```python
from build123d import *

# Parameters (mm, degrees)
F0_R     = 1.5875
F1_DEPTH = 12.7


with BuildPart() as f1:
    # F0 (on Front) → F1 (new body)
    with BuildSketch(Plane.XZ):
        with BuildLine():
            Line((-12.238163, 28.612093), (-55.574305, 28.462326))
            ThreePointArc((-55.574305, 28.462326), (-59.292865, 24.743766), (-55.574305, 21.025206))
            Line((-55.574305, 21.025206), (-12.224796, 20.875369))
            ThreePointArc((-12.224796, 20.875369), (-8.343011, 24.73708), (-12.211425, 28.612186))
            ThreePointArc((-12.211425, 28.612186), (-12.224794, 28.612162), (-12.238163, 28.612093))
        make_face()
        with Locations((-55.574305, 24.743766)):
            Circle(F0_R, mode=Mode.SUBTRACT)
        with Locations((-12.211425, 24.743766)):
            Circle(F0_R, mode=Mode.SUBTRACT)
    extrude(amount=F1_DEPTH)


solid = f1.part
```
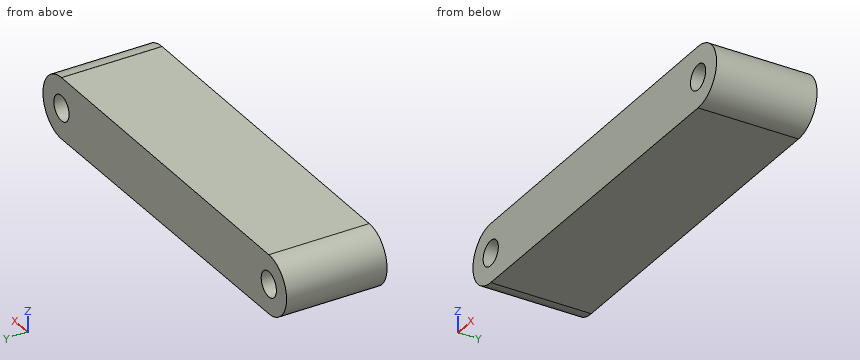
Source: CAD feature listing. Evaluate the final solid. Frame: model axes, mm. Give positions to 0.01 mm unless a question says otherwise; leave off trailing zeros. Order: outer loops, then holes, each group sorted by start corner. A loop starts at its lowest first (then second) coordinate and runs counter-clockwise, first axis right, second up.
(1) Contact query for flat-ended pins moving along their axis: P1, Ø4, axis at y = -9, z = 22, coming from the +X side; P2, Ø1.9, axis at x = -55.57, z = 24.74, coming from the +Y side; P3, Ø1.5, axis at y = -3.5, z = 22.5, coming from the +X side; P4, Ø1, axis at y = -7, z = 28, coming from the -X side. Output: stop coordinate, or through.
(2) Section query A-A (z = 23.75). Return the cut outline in (x, y), plus the area to 3 significant figures.
(3) Section query D-D (z = 28). Return the cut outline in (x, y).
(4) Section query B-B (y = -4.5). State how many separate pieces and enclosed holes the cut face has, plus the area to 3 significant figures.
(5) Material intervals for line 1 along X through (y, z) = (-6.5, 24.75); line 2 along X through (y, z) = (-9.5, 26); line 3 along Z through (x, y) = (-11, -7), sorted ascending.
(6) Section query C-C (x = -32.5). Return the cut outline in (y, z), plus the area to 3 significant figures.
Outcome:
1. P1: stops at x = -8.42
1. P2: passes through
1. P3: stops at x = -8.64
1. P4: stops at x = -58.07
2. outline: (-59.16, -12.7) - (-56.81, -12.7) - (-56.81, 0) - (-59.16, 0) - close; (-54.34, -12.7) - (-13.45, -12.7) - (-13.45, 0) - (-54.34, 0) - close; (-10.97, -12.7) - (-8.47, -12.7) - (-8.47, 0) - (-10.97, 0) - close
2. area: 581 mm2
3. outline: (-57.37, -12.7) - (-10.12, -12.7) - (-10.12, 0) - (-57.37, 0) - close
4. separate pieces: 1
4. enclosed holes: 2
4. area: 358 mm2
5. line 1: x = -59.29 to -57.16, -53.99 to -13.8, -10.62 to -8.34
5. line 2: x = -59.07 to -56.54, -54.6 to -13.18, -11.24 to -8.55
5. line 3: z = 21.07 to 23.72, 25.77 to 28.42
6. outline: (-12.7, 20.95) - (0, 20.95) - (0, 28.54) - (-12.7, 28.54) - close
6. area: 96.5 mm2
